Autodesk Inventor part; units mm, degrees
ref_plane "YZ Plane" through (0, 0, 0) normal (1, 0, 0) x (0, 1, 0)
ref_plane "XZ Plane" through (0, 0, 0) normal (0, 1, 0) x (-1, 0, 0)
ref_plane "XY Plane" through (0, 0, 0) normal (0, 0, 1) x (1, 0, 0)
sketch "Sketch1" plane through (0, 0, 0) normal (1, 0, 0) x (0, 1, 0)
  line L0 (-11.1125, -4.7625) -> (11.1125, -4.7625)
  line L1 (11.1125, -4.7625) -> (11.1125, 4.7625)
  line L2 (11.1125, 4.7625) -> (-11.1125, 4.7625)
  line L3 (-11.1125, 4.7625) -> (-11.1125, -4.7625)
  line L4 (-11.1125, -4.7625) -> (11.1125, 4.7625) construction
  line L5 (11.1125, -4.7625) -> (-11.1125, 4.7625) construction
  circle A0 centre (5.5563, 0) radius 2.1082
  circle A1 centre (-5.5562, 0) radius 2.1082
  point P0 (0, 0)
  point P1 (-11.1125, 0)
  dimension "d0" = 9.525
  dimension "d1" = 22.225
  dimension "d2" = 4.2164
  dimension "d3" = 4.2164
  dimension "d4" = 5.5563
  dimension "d5" = 5.5563
extrude "Extrusion1" add sketch "Sketch1" along normal blind 12.7
sketch "Sketch2" plane through (12.7, 0, 0) normal (1, 0, 0) x (0, 0, -1)
  circle A0 centre (0, 5.5563) radius 2.1082
  line L0 (0, 10.5972) -> (4.3656, 8.0767)
  line L1 (4.3656, 8.0767) -> (4.3656, 3.0358)
  line L2 (4.3656, 3.0358) -> (0, 0.5153)
  line L3 (0, 0.5153) -> (-4.3656, 3.0358)
  line L4 (-4.3656, 3.0358) -> (-4.3656, 8.0767)
  line L5 (-4.3656, 8.0767) -> (0, 10.5972)
  circle A1 centre (0, -5.5562) radius 2.1082
  line L6 (0, -0.5153) -> (4.3656, -3.0358)
  line L7 (4.3656, -3.0358) -> (4.3656, -8.0767)
  line L8 (4.3656, -8.0767) -> (0, -10.5972)
  line L9 (0, -10.5972) -> (-4.3656, -8.0767)
  line L10 (-4.3656, -8.0767) -> (-4.3656, -3.0358)
  line L11 (-4.3656, -3.0358) -> (0, -0.5153)
  line L12 (4.7625, 11.1125) -> (-4.7625, 11.1125)
  line L13 (-4.7625, 11.1125) -> (-4.7625, -11.1125)
  line L14 (-4.7625, -11.1125) -> (4.7625, -11.1125)
  line L15 (4.7625, -11.1125) -> (4.7625, 11.1125)
  circle A2 centre (0, 5.5563) radius 2.1082
  circle A3 centre (0, -5.5562) radius 2.1082
  line L16 (-4.3656, 8.0767) -> (4.3656, 8.0767)
  line L17 (4.3656, 8.0767) -> (4.3656, 13.7838)
  line L18 (4.3656, 13.7838) -> (-4.3656, 13.7838)
  line L19 (-4.3656, 13.7838) -> (-4.3656, 8.0767)
  line L20 (-4.3656, -8.0767) -> (4.3656, -8.0767)
  line L21 (4.3656, -8.0767) -> (4.3656, -13.1177)
  line L22 (4.3656, -13.1177) -> (-4.3656, -13.1177)
  line L23 (-4.3656, -13.1177) -> (-4.3656, -8.0767)
  point P0 (-4.3656, 11.1125)
  point P1 (-4.3656, -11.1125)
  point P2 (4.3656, -11.1125)
  point P3 (4.3656, 11.1125)
  dimension "d10" = 4.3656
  dimension "d11" = 4.3656
extrude "Extrusion2" add sketch "Sketch2" along normal blind 6.35 contours L17 L12 L15 L14 L21 L7 L6 L11 L10 L23 L13 L19 L4 L3 L2 L1
sketch "Sketch3" plane through (19.05, 0, 0) normal (1, 0, 0) x (0, 0, -1)
  line L0 (-4.7625, 11.1125) -> (-4.7625, -11.1125)
  line L1 (4.7625, -11.1125) -> (-4.7625, -11.1125)
  line L2 (-4.7625, -11.1125) -> (-4.7625, 11.1125)
  line L3 (-4.7625, 11.1125) -> (4.7625, 11.1125)
  line L4 (4.7625, 11.1125) -> (4.7625, -11.1125)
  line L5 (4.7625, -11.1125) -> (-4.7625, 11.1125) construction
  line L6 (-4.7625, -11.1125) -> (4.7625, 11.1125) construction
  point P0 (0, 0)
extrude "Extrusion3" add sketch "Sketch3" along normal blind 19.05
sketch "Sketch4" plane through (0, 11.1125, 4.7625) normal (0, 1, 0) x (1, 0, 0)
  circle A0 centre (25.4, 4.7625) radius 2.1082
  line L0 (38.1, 9.525) -> (38.1, 0)
  line L1 (0, 9.525) -> (0, 0)
  point P0 (0, 4.7625)
  dimension "d16" = 4.2164
  dimension "d25" = 25.4
extrude "Extrusion4" cut sketch "Sketch4" against normal blind 25.4
fillet "Fillet1" radius 0.7937 4 edges at (38.1, 0, -4.7625) (38.1, 11.1125, 0) (38.1, 0, 4.7625) (38.1, -11.1125, 0)
fillet "Fillet2" radius 0.7937 8 edges at (37.8675, 10.88, -4.53) (18.6531, 11.1125, -4.7625) (37.8675, 10.88, 4.53) (18.6531, 11.1125, 4.7625) (37.8675, -10.88, -4.53) (18.6531, -11.1125, -4.7625) (37.8675, -10.88, 4.53) (18.6531, -11.1125, 4.7625)
fillet "Fillet3" radius 0.7937 8 edges at (0, 10.88, 4.53) (0, 0, 4.7625) (0, -10.88, 4.53) (0, -11.1125, 0) (0, -10.88, -4.53) (0, 0, -4.7625) (0, 10.88, -4.53) (0, 11.1125, 0)
fillet "Fillet4" radius 0.3969 2 edges at (23.2918, 11.1125, 0) (23.2918, -11.1125, 0)
fillet "Fillet5" radius 0.3969 2 edges at (0, 3.4481, 0) (0, -7.6644, 0)
properties part number ".5x1 Tube Stock Insert" material "PBT Plastic"
Model file for the job. Use its own axes, mm. A direction names the side the tool comes from. Round coordinates to 2 decimals unless told otherwise and drop trailing zeros. Order: outer loops, then holes, each group sorted by start corner. A loop starts at its lowest first (then second) coordinate and runs counter-clockwise, first axis right, second up. Notation, with made-up numbers: M 50,31 L 95,31 A22 cw 95,69 Z; hole C 44.5,-27 d11. An arc over 180 degrees is marked long. Write each question's results on one line, items separated by ' | '. Start each with the question number.
(1) Drop a flat-ended pin along its axis: pin 1 (2 mm diameter, centred on x = 15, z = 0, fed in from -Y). Give the stop position or say it passes through.
(2) Probe probe 1 along X at (y, z) = (9.25, -4); probe 2 along Z at (x, y) = (18, -5.25); probe 3 along Z at (x, y) = (5.5, -5.5). List the from-to ranges inside material, lowest first. Write a range as from..to.
(3) Saw through at A-A, the plane y = 8.75. Give the cut face in (x, z).
(4) Saw through at B-B, the plane x = 25.4. Give the cut face in (y, z), then the cut area to 3 significant figures.
(5) Saw through at D-D, the plane z = 3.25. Give the cut face in (x, y), then the cut area to 3 significant figures.
(6) Which spindle directions (+Z, -Z, +X, -X, +Y, -Y) get a long thin tool onto all of the face, cutting with end or side? Do faces 1 (the face through (0, 0, 0)), 2 (the face through (12.7, -8, 0)), 3 (the face through (6.462, -3.545, -0.633)), 4 (the face through (15.831, 1.758, 2.152)). Say none if no direction does.
(7) Two-plate mould, pull along Z, no slides. Class faces 5 (the face through (19, 0, 4.762)), 6 (the face through (19, 0, -4.762)), 7 (the face through (7, -11.112, 0)), 8 (the face through (15.83, 1.79, -2.21)): pulls with the +Z half, pulls with the -Z half, needs draft (parallel to the pull), parting line crosses it, or undercut.
(8) Saw through at C-C, the plane x = 3. Give the cut face in (y, z), then the cut area to 3 significant figures.
Established:
1) pin 1: stops at y = -1.09
2) probe 1: x = 0..12.7, 19.05..38.1 | probe 2: z = -4.76..-4.37, 4.37..4.76 | probe 3: z = -4.76..-2.11, 2.11..4.76
3) outline: M 0,-3.97 A0.79 ccw 0.79,-4.76 L 37.31,-4.76 A0.79 ccw 38.1,-3.97 L 38.1,3.97 A0.79 ccw 37.31,4.76 L 0.79,4.76 A0.79 ccw 0,3.97 Z; hole M 12.7,-4.37 L 19.05,-4.37 L 19.05,4.37 L 12.7,4.37 Z; hole C 25.4,0 d4.22
4) outline: M -11.11,-3.97 A0.79 ccw -10.32,-4.76 L 10.32,-4.76 A0.79 ccw 11.11,-3.97 L 11.11,-2.51 A0.4 ccw 10.72,-2.11 L -10.72,-2.11 A0.4 ccw -11.11,-2.51 Z; M -11.11,2.51 A0.4 ccw -10.72,2.11 L 10.72,2.11 A0.4 ccw 11.11,2.51 L 11.11,3.97 A0.79 ccw 10.32,4.76 L -10.32,4.76 A0.79 ccw -11.11,3.97 Z | area: 117 mm^2
5) outline: M 0,-10.32 A0.79 ccw 0.79,-11.11 L 12.7,-11.11 L 12.7,-2.39 L 19.05,-2.39 L 19.05,-11.11 L 37.31,-11.11 A0.79 ccw 38.1,-10.32 L 38.1,10.32 A0.79 ccw 37.31,11.11 L 19.05,11.11 L 19.05,2.39 L 12.7,2.39 L 12.7,11.11 L 0.79,11.11 A0.79 ccw 0,10.32 Z | area: 735 mm^2
6) face 1: +Z, -Z, -X, +Y, -Y | face 2: -Y | face 3: -X | face 4: +Y
7) face 5: pulls with the +Z half | face 6: pulls with the -Z half | face 7: needs draft | face 8: undercut
8) outline: M -11.11,-3.97 A0.79 ccw -10.32,-4.76 L 10.32,-4.76 A0.79 ccw 11.11,-3.97 L 11.11,3.97 A0.79 ccw 10.32,4.76 L -10.32,4.76 A0.79 ccw -11.11,3.97 Z; hole C -5.56,0 d4.22; hole C 5.56,0 d4.22 | area: 183 mm^2
